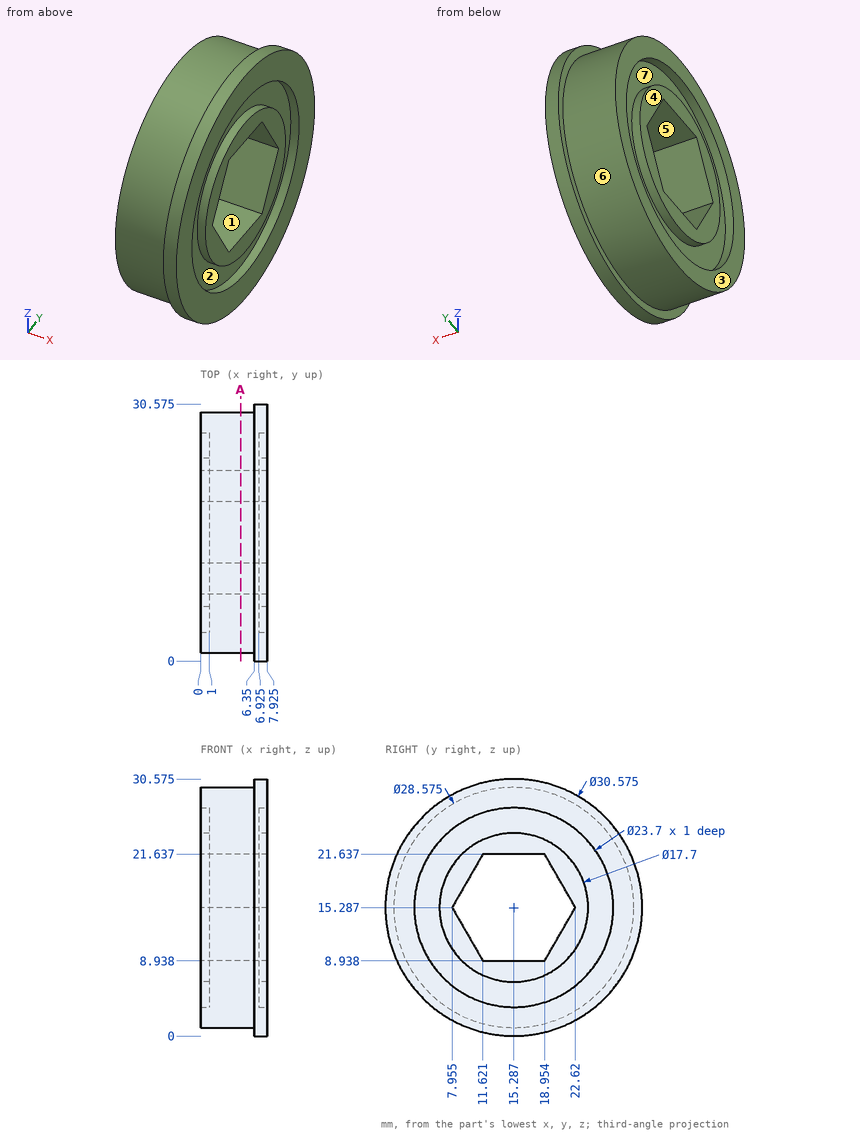
Here's the drawing with two shaded views (mm, measured from the low corner). I have some questions. A direction names the side the tool comes from. Coordinates: 2 decimals unless noted, no trailing zeros. Loops run counter-clockwise (first coordinate to the right, second up) from the corner with the lowest first, then second, coordinate; pieces in that order, holes last. Notation, with made-up numbers: (79.5, -8.5) -> (131.5, -8.5) arc R22 ccw to (131.5, 3.5) -> close; hole circle Ø3 at (5.25, 22). An arc over 180 degrees is marked (long way). Put each result on its own line as item: value. Start each with the question number.
Q1. If I drill on line 1 (X direction, y = 9, z = 6) (1 decimal); line 2 (Z direction, x = 1.25, y = 22) (1 decimal); line 3 (Y direction, x = 5.25, z = 15.5) (1 decimal), over which ranges is the centre line in solid material (lowest first)? Write a range as [from, to].
Q2. I'm going to push flat-ended pins straight in: P1, Ø1.5, axis at x = 2.5, y = 17, coming from the +Z side; P2, Ø3, axis at x = 1.5, z = 20, coming from the +Y side; P3, Ø2, axis at x = 2.5, y = 15.5, coming from the -Z side. Where does each tip first touch, or does it pass through?
Q3. Thinking about a two-plate mould opening in Y: for the marked faces 4, 5, 6 and 7, which applies, pulls with the +Y half, pulls with the -Y half, needs draft (parallel to the pull), parting line crosses it, or undercut?
Q4. I want a section at A-A (x = 4.75). Write out the boundary of the cut face in (y, z) (1 decimal).
Q5. For the marked faces 1, 2 and 3, which set-ups out of +Z, -Z, +X, -X, +Y, -Y let a thin tool reach every point of the face, with its end or its side?
Taken from the geometry:
1. line 1: x = [1, 6.9]
1. line 2: z = [2.7, 14.2], [16.4, 27.9]
1. line 3: y = [1, 8.1], [22.5, 29.6]
2. P1: stops at z = 29.54
2. P2: stops at y = 29.21
2. P3: stops at z = 1
3. face 4: needs draft
3. face 5: undercut
3. face 6: parting line crosses it
3. face 7: undercut
4. outline: circle Ø28.6 at (15.3, 15.3); hole (8, 15.3) -> (11.6, 8.9) -> (19, 8.9) -> (22.6, 15.3) -> (19, 21.6) -> (11.6, 21.6) -> close
5. face 1: +X, -X
5. face 2: +X
5. face 3: +Z, -Z, -X, +Y, -Y
